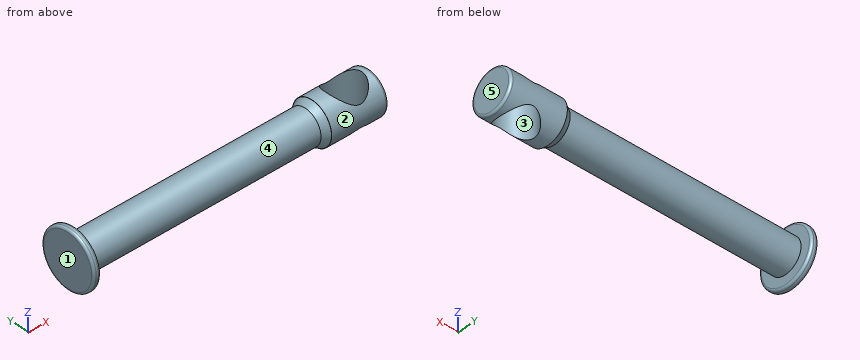
```python
from build123d import *

# Parameters (mm, degrees)
CHAMFER1_SIZE           = 3
CHAMFER1_SIZE2          = 1.732050808
CUT_EXTRUDE1_DEPTH      = 135.169668703
CUT_EXTRUDE1_DEPTH_BACK = 135.169668703
SKETCH2_R               = 8
FILLET1_R               = 1


with BuildPart() as part:
    # Sketch1 → Revolve1 (revolve)
    with BuildSketch(Plane(origin=(0, 0, 0), x_dir=(1, 0, 0), z_dir=(0, 1, 0))):
        Polygon((0, 0), (0, 12.5), (3, 12.5), (3, 7.5), (108, 7.5), (108, 9.35), (133, 9.35), (133, 0), align=None)
    revolve(axis=Axis((133, 0, 0), (-1, 0, 0)))

    # Chamfer1
    chamfer1_edges = [part.edges().sort_by_distance(p)[0] for p in [
        (108, 0, 7.5),
    ]]
    chamfer1_side = [part.faces().sort_by_distance(p)[0] for p in [
        (55.5, 0, 7.5),
    ]]
    chamfer(chamfer1_edges, length=CHAMFER1_SIZE, length2=CHAMFER1_SIZE2, reference=chamfer1_side[0])

    # Sketch2 → Cut-Extrude1 (cut, two sides: drawn at the far end of the back side and taken through both)
    with BuildSketch(Plane.XY.offset(-CUT_EXTRUDE1_DEPTH_BACK)):
        with Locations((122, 0)):
            Circle(SKETCH2_R)
    extrude(amount=CUT_EXTRUDE1_DEPTH + CUT_EXTRUDE1_DEPTH_BACK, mode=Mode.SUBTRACT)

    # Fillet1
    fillet1_edges = [part.edges().sort_by_distance(p)[0] for p in [
        (133, 0, 9.35),
        (3, 0, 12.5),
        (0, 0, 12.5),
    ]]
    fillet(fillet1_edges, radius=FILLET1_R)


solid = part.part
```
The listing builds one solid part. Answer for the finished solid, in the listing's coordinates (mm). Face numbers are marked on the shaded views. A direction names the side the tool comes from. Round coordinates to 2 decimals unless told otherwise and drop trailing zeros. Loops run counter-clockwise (first coordinate to the right, second up) from the corner with the lowest first, then second, coordinate; pieces in that order, holes last. Notation, with made-up numbers: (-11.5, 7.25) - (3.5, 7.25) arc R31 ccw to (3.5, 40.25) - close; hole circle Ø7 at (-20, 20). An arc over 180 degrees is marked (long way). Use one line per item in the form item = value. Start each with the question number.
1. Consider line 1 (X direction, y = 0, z = 2); line 2 (X direction, y = 6, z = -6.25); line 3 (X direction, y = 0.5, z = 9). Determine where each line is inside the solid, lowest interval first. Write a range as [from, to].
2. For a pull along Y with two mould halves and no side action, classify the marked faces 3, 4 and 5 as pulls with the +Y half, pulls with the -Y half, needs draft (parallel to the pull), parting line crosses it, or undercut.
3. The part is cut by section D-D on x = 56. Determine the outline of the cut face in (y, z).
4. The part is cut by section B-B on z = 0. Determine the outline of the cut face in (x, y).
5. The part is cut by section A-A on y = 0. Determine the outline of the cut face in (x, z), then the cut area to 3 significant figures.
6. Given pin 1 Ø4 at (x, z) = (30, 1) entering from +Y; pin 2 Ø12 at (x, y) = (29, 0.5) entering from -Z; pin 3 Ø8 at (x, z) = (64, -9) entering from -Y; pin 4 Ø3 at (x, y) = (103.5, -10) entering from +Z, each flat-ended and moving along its own axis, determine where each tip first touches the part or whether it passes through.
7. A tool of negligible diameter and unlimited length cuts with its end or side. For the marked faces 1 and 2, from which of +Z, -Z, +X, -X, +Y, -Y can it reach the whole face along a straight path? Write none if from no direction.
8. The part is cut by section C-C on x = 118.5. Determine the outline of the cut face in (y, z), then the cut area to 3 significant figures.
Geometry check:
q1.line_1 = [0, 114], [130, 133]
q1.line_2 = [0, 3], [107.02, 116.71], [127.29, 132.95]
q1.line_3 = [0, 3], [107.62, 114.02], [129.98, 132.75]
q2.face_3 = undercut
q2.face_4 = parting line crosses it
q2.face_5 = needs draft
q3.outline = circle Ø15 at (0, 0)
q4.outline = (0, -11.5) arc R1 ccw to (1, -12.5) - (2, -12.5) arc R1 ccw to (3, -11.5) - (3, -7.5) - (105, -7.5) - (108, -9.23) - (108, -9.35) - (132, -9.35) arc R1 ccw to (133, -8.35) - (133, 8.35) arc R1 ccw to (132, 9.35) - (108, 9.35) - (108, 9.23) - (105, 7.5) - (3, 7.5) - (3, 11.5) arc R1 ccw to (2, 12.5) - (1, 12.5) arc R1 ccw to (0, 11.5) - close; hole circle Ø16 at (122, 0)
q5.outline = (0, -11.5) arc R1 ccw to (1, -12.5) - (2, -12.5) arc R1 ccw to (3, -11.5) - (3, -7.5) - (105, -7.5) - (108, -9.23) - (108, -9.35) - (114, -9.35) - (114, 9.35) - (108, 9.35) - (108, 9.23) - (105, 7.5) - (3, 7.5) - (3, 11.5) arc R1 ccw to (2, 12.5) - (1, 12.5) arc R1 ccw to (0, 11.5) - close; (130, -9.35) - (132, -9.35) arc R1 ccw to (133, -8.35) - (133, 8.35) arc R1 ccw to (132, 9.35) - (130, 9.35) - close
q5.area = 1,820 mm^2
q6.pin_1 = 7.5
q6.pin_2 = -7.5
q6.pin_3 = -5.59
q6.pin_4 = through
q7.face_1 = +Z, -Z, -X, +Y, -Y
q7.face_2 = +X
q8.outline = (-7.19, -5.97) - (-7.19, 5.97) arc R9.35 ccw to start; (7.19, -5.97) arc R9.35 ccw to (7.19, 5.97) - close
q8.area = 35.2 mm^2
